from build123d import *

# Parameters (mm, degrees)
SKETCH_1_R      = 45
EXTRUDE_1_DEPTH = 8


with BuildPart() as part:
    # 草图1 → 凸台-拉伸1 (new body)
    with BuildSketch(Plane(origin=(0, 0, 0), x_dir=(0, 0, -1), z_dir=(1, 0, 0))):
        Polygon((70, 98), (-620, 98), (-620, -77.5), (-599.5, -98), (70, -98), align=None)
        Circle(SKETCH_1_R, mode=Mode.SUBTRACT)
    extrude(amount=EXTRUDE_1_DEPTH)


solid = part.part
Could you check a few things on this model? Use its own coordinates, in mm. Give positions to 0.01 mm unless a question says otherwise; leave off trailing zeros. Write each loop counter-clockwise with the first axis right and the second up, starting at its lowest first coordinate (ties: lowest second). Pieces come first, ordered by that corner, then holes. Notation, with made-up numbers: (88.25, -15) -> (97.25, -15) arc R27 cw to (97.25, 19) -> close; hole circle Ø11 at (11.5, -36). An arc over 180 degrees is marked (long way). Write each question's results on one line, items separated by ' | '. Start each with the question number.
Q1. Suppose I cut it at B-B, the plane y = 0. List the corners of the cut face in (x, z) for me.
Q2. I need wall thicknesses on probe 1 along Y at (x, z) = (4.25, 0); probe 2 along Z at (x, y) = (1.25, -21.5); probe 3 along Y at (x, z) = (1.25, -15.5). Which ranges of each line are inside material? Lowest first, please.
Q3. We'd pull the mould along Z, two halves only. Please class faces 1 (the face through (3.9, -87.6, 609.9)), 2 (the face through (0, 1, 280)), 3 (the face through (3.944, -39.923, -20.765)): +Z half, -Z half, draft (parallel to the pull), parting line (faces both ways), or undercut.
Q4. Suppose I cut it at C-C, the plane x = 6. List the corners of the cut face in (y, z) for me, and give its area (3 significant figures).
Q5. Suppose I cut it at A-A, the plane z = 0. List the corners of the cut face in (x, y) for me, and give its area (3 significant figures).
Outcome:
1) outline: (0, -70) -> (8, -70) -> (8, -45) -> (0, -45) -> close; (0, 45) -> (8, 45) -> (8, 620) -> (0, 620) -> close
2) probe 1: -98 to -45, 45 to 98 | probe 2: -70 to -39.53, 39.53 to 620 | probe 3: -98 to -42.25, 42.25 to 98
3) face 1: +Z half | face 2: draft | face 3: undercut
4) outline: (-98, -70) -> (98, -70) -> (98, 620) -> (-77.5, 620) -> (-98, 599.5) -> close; hole circle Ø90 at (0, 0) | area: 129,000 mm2
5) outline: (0, -98) -> (8, -98) -> (8, -45) -> (0, -45) -> close; (0, 45) -> (8, 45) -> (8, 98) -> (0, 98) -> close | area: 848 mm2
